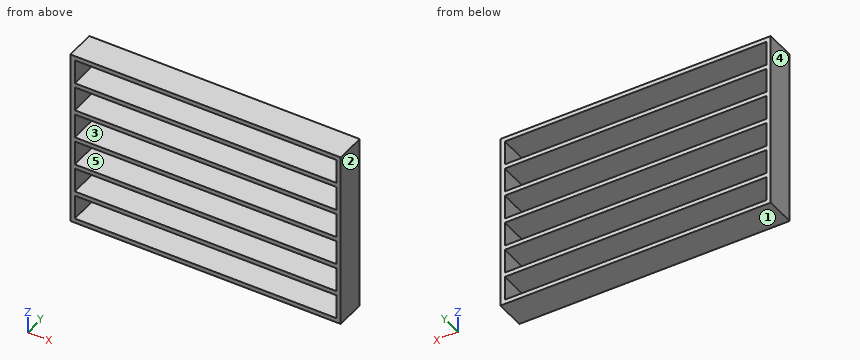
from build123d import *

# Parameters (mm, degrees)
F0_W     = 1520
F0_H     = 1000
F1_DEPTH = 170
F2_W     = 1470
F2_H     = 137.5
F3_DEPTH = 170


with BuildPart() as f1:
    # F0 (on Front) → F1 (new body)
    with BuildSketch(Plane.XZ):
        Rectangle(F0_W, F0_H)
    extrude(amount=-F1_DEPTH)

    # F2 (on face) → F3 (cut, through all)
    with BuildSketch(Plane.XZ):
        with Locations((0, 406.25)):
            Rectangle(F2_W, F2_H)
        with Locations((0, 243.75)):
            Rectangle(F2_W, F2_H)
        with Locations((0, 81.25)):
            Rectangle(F2_W, F2_H)
        with Locations((0, -81.25)):
            Rectangle(F2_W, F2_H)
        with Locations((0, -243.75)):
            Rectangle(F2_W, F2_H)
        Polygon((-735, -337.5), (-735, -475), (735, -475), (735, -425), (735, -337.5), align=None)
    extrude(amount=-F3_DEPTH, mode=Mode.SUBTRACT)


solid = f1.part
Could you check a few things on this model? Use its own coordinates, in mm. Face numbers are marked on the shaded views. A direction names the side the tool comes from. Round coordinates to 2 decimals unless told otherwise and drop trailing zeros. Order: outer loops, then holes, each group sorted by start corner. A loop starts at its lowest first (then second) coordinate and runs counter-clockwise, first axis right, second up.
Q1. Which directions (+Z, -Z, +X, -X, +Y, -Y) give clear straight access to the entire face, cutting with the end or side of a thin tool? Please do the marked faces 4 and 5.
Geometry says:
face 4: +Z, -Z, -X, +Y, -Y
face 5: +Y, -Y
Q2. Thinking about a two-plate mould opening in X: for the marked faces 1, 2 and 3, which applies, released by +X, released by -X, zero draft, split by the parting line, or undercut?
Geometry says:
face 1: zero draft
face 2: released by +X
face 3: undercut
Q3. Imagine slicing it at C-C, the plane y = 138.5. List the corners of the cut face in (x, z) for me, then the cut area to 3 significant figures.
Geometry says:
outline: (-760, -500) - (760, -500) - (760, 500) - (-760, 500) - close; hole (-735, -475) - (735, -475) - (735, -337.5) - (-735, -337.5) - close; hole (-735, -312.5) - (735, -312.5) - (735, -175) - (-735, -175) - close; hole (-735, -150) - (735, -150) - (735, -12.5) - (-735, -12.5) - close; hole (-735, 12.5) - (735, 12.5) - (735, 150) - (-735, 150) - close; hole (-735, 175) - (735, 175) - (735, 312.5) - (-735, 312.5) - close; hole (-735, 337.5) - (735, 337.5) - (735, 475) - (-735, 475) - close
area: 307,000 mm2
Q4. Imagine slicing it at B-B, the plane z = 406.5. List the corners of the cut face in (x, y) for me.
Geometry says:
outline: (-760, 0) - (-735, 0) - (-735, 170) - (-760, 170) - close; (735, 0) - (760, 0) - (760, 170) - (735, 170) - close
Q5. Imagine slicing it at A-A, the plane x = 375.5. List the corners of the cut face in (y, z) for me.
Geometry says:
outline: (0, -500) - (170, -500) - (170, -475) - (0, -475) - close; (0, -337.5) - (170, -337.5) - (170, -312.5) - (0, -312.5) - close; (0, -175) - (170, -175) - (170, -150) - (0, -150) - close; (0, -12.5) - (170, -12.5) - (170, 12.5) - (0, 12.5) - close; (0, 150) - (170, 150) - (170, 175) - (0, 175) - close; (0, 312.5) - (170, 312.5) - (170, 337.5) - (0, 337.5) - close; (0, 475) - (170, 475) - (170, 500) - (0, 500) - close
Q6. Please list where this line runs through material, in increasing order: probe 1 along X at (y, z) = (11, -277.5).
Geometry says:
probe 1: x = -760 to -735, 735 to 760
